Answer from the drawing. Dimensions are ordinates in mm from the lowest x, y and z of the part. Round coordinates to 2 decimals unless told otherwise and drop trailing zeros. Write each loop counter-clockwise with the first axis right and the second up, starting at its lowest first coordinate (ties: lowest second). Pieces come first, ordered by that corner, then holes. Notation, with made-up numbers: (32.5, -7.5) - (52.5, -7.5) arc R28 cw to (52.5, 20.5) - close; hole circle Ø4 at (20.25, 12). An arc over 180 degrees is marked (long way). Answer in a Markdown table with one row per item.
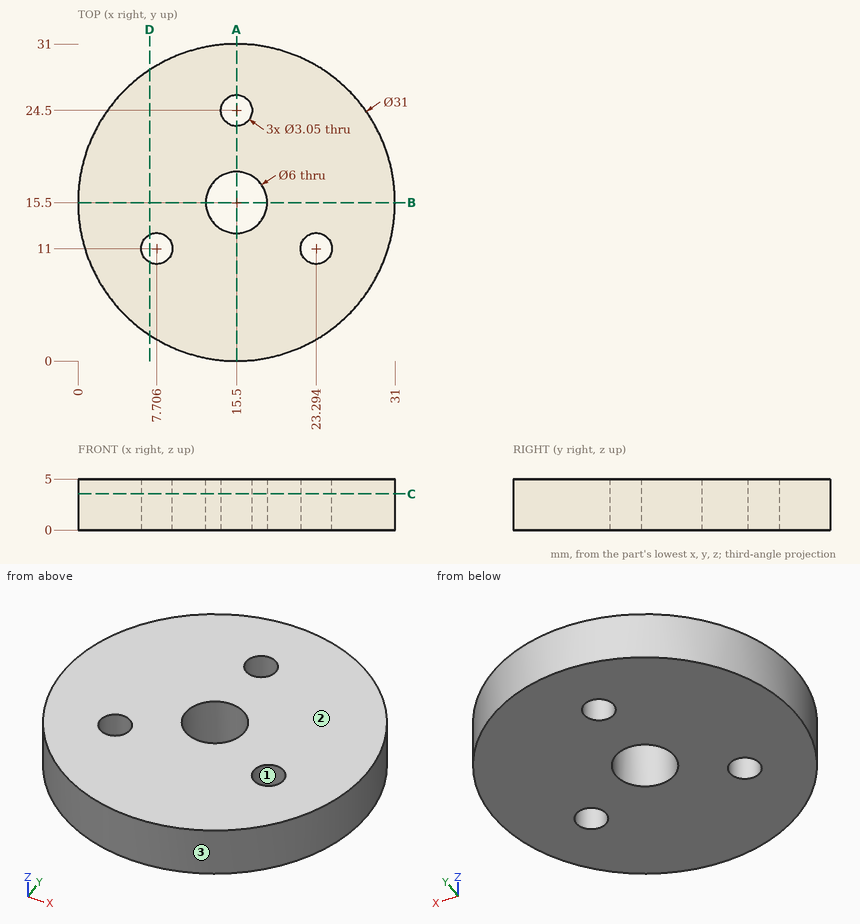
(1) Find the intervals of material crossed by line 1 (Y direction, x = 15.5, z = 4.15) (3 decimals); line 2 (X direction, y = 11.5, z = 1.65) (1 decimal); line 3 (X direction, y = 24.5, z = 2.55) (1 decimal), in increasing order.
Checked values:
| item | result |
|---|---|
| line 1 | y = 0 to 12.5, 18.5 to 22.975, 26.025 to 31 |
| line 2 | x = 0.5 to 6.3, 9.1 to 21.9, 24.7 to 30.5 |
| line 3 | x = 2.9 to 14, 17 to 28.1 |
(2) For a pull along X with two mould halves and no side action, classify the marked faces 1, 2 and 3 as pulls with the +X half, pulls with the -X half, needs draft (parallel to the pull), parting line crosses it, or undercut.
Checked values:
| item | result |
|---|---|
| face 1 | undercut |
| face 2 | needs draft |
| face 3 | parting line crosses it |
(3) Flat-ended cylindrical pins translate along their axes: pin 1 (4 mm diameter, centred on x = 23, y = 11, fed in from +Z); pin 2 (1 mm diameter, centred on y = 25.5, z = 2.5, fed in from -X); pin 3 (2 mm diameter, centred on y = 11, z = 2, fed in from -X). Find the tip coordinate at first contact, or state that the pin passes through.
Checked values:
| item | result |
|---|---|
| pin 1 | stops at z = 5 |
| pin 2 | stops at x = 3.25 |
| pin 3 | stops at x = 0.4 |
(4) Section A-A (x = 15.5) is taken. Give the vertices of the cut face in (y, z) (3 decimals).
Checked values:
| item | result |
|---|---|
| outline | (0, 0) - (12.5, 0) - (12.5, 5) - (0, 5) - close; (18.5, 0) - (22.975, 0) - (22.975, 5) - (18.5, 5) - close; (26.025, 0) - (31, 0) - (31, 5) - (26.025, 5) - close |
(5) Section B-B (y = 15.5) is taken. Give the vertices of the cut face in (x, z).
Checked values:
| item | result |
|---|---|
| outline | (0, 0) - (12.5, 0) - (12.5, 5) - (0, 5) - close; (18.5, 0) - (31, 0) - (31, 5) - (18.5, 5) - close |
(6) Section C-C (z = 3.55) is taken. State how many separate pieces and enclosed holes the cut face has, and give its area (3 significant figures).
Checked values:
| item | result |
|---|---|
| separate pieces | 1 |
| enclosed holes | 4 |
| area | 705 mm2 |
(7) Section D-D (x = 7) is taken. Give the vertices of the cut face in (y, z), and give its area (3 significant figures).
Checked values:
| item | result |
|---|---|
| outline | (2.54, 0) - (9.65, 0) - (9.65, 5) - (2.54, 5) - close; (12.35, 0) - (28.46, 0) - (28.46, 5) - (12.35, 5) - close |
| area | 116 mm2 |
